Could you check a few things on this drawing? It's one solid part, dimensions in mm from its lowest x, y, z. A direction names the side the tool comes from. Coordinates: 2 decimals unless noted, no trailing zeros. Order: outer loops, then holes, each group sorted by start corner. A loop starts at its lowest first (then second) coordinate and runs counter-clockwise, first axis right, second up. Notation, with made-up numbers: (57.25, 73) - (111.25, 73) arc R32 cw to (111.25, 111) - close; hole circle Ø3 at (69, 32.25). An arc over 180 degrees is marked (long way). Return JSON: item names as keys, results as strings. Group by question number.
1) Imagine slicing it at A-A (y = 18). Write out the boundary of the cut face in (x, z).
2) For pin 1 Ø4 at (y, z) = (6, 75) entering from -X; pin 2 Ø3 at (x, y) = (9.5, 23) entering from -Z; pin 3 Ø1.2 at (x, y) = (9.5, 13.5) entering from -Z, each with a flat end and sliding along its axis, tell me the tip position at first contact or that it passes through.
3) If I drill on line 1 along Z through (x, y) = (28.5, 18.5); line 2 along X through (y, z) = (13, 24); line 3 along Z through (x, y) = (23, 21), over which ranges is the centre line in solid material (lowest first)?
4) Which directions (+Z, -Z, +X, -X, +Y, -Y) give clear straight access to the entire face, cutting with the end or side of a thin tool? Please do the marked faces 1 and 2.
5) Imagine slicing it at D-D (x = 4). Write out the boundary of the cut face in (y, z), and give its area (3 significant figures).
6) Imagine slicing it at B-B (z = 68). Write out the boundary of the cut face in (x, y).
7) Imagine slicing it at C-C (y = 27.5). Write out the boundary of the cut face in (x, z).
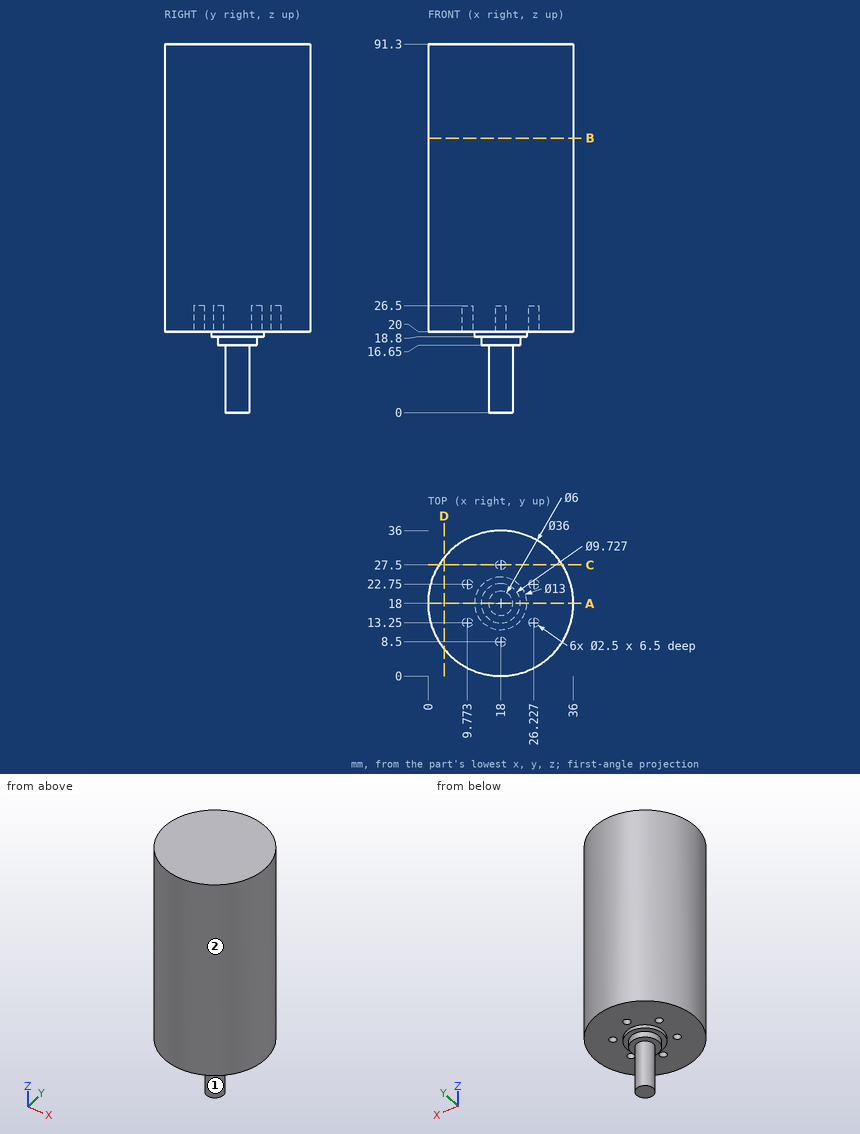
Calculated:
{
 "1": {"outline": "(0, 20) - (11.5, 20) - (11.5, 18.8) - (13.14, 18.8) - (13.14, 16.65) - (15, 16.65) - (15, 0) - (21, 0) - (21, 16.65) - (22.86, 16.65) - (22.86, 18.8) - (24.5, 18.8) - (24.5, 20) - (36, 20) - (36, 91.3) - (0, 91.3) - close"},
 "2": {"pin 1": "x = 3.03", "pin 2": "z = 20", "pin 3": "z = 26.5"},
 "3": {"line 1": "20 to 91.3", "line 2": "0.71 to 8.55, 11 to 25, 27.45 to 35.29", "line 3": "18.8 to 91.3"},
 "4": {"face 1": "-Z", "face 2": "+Z, -Z"},
 "5": {"outline": "(6.69, 20) - (29.31, 20) - (29.31, 91.3) - (6.69, 91.3) - close", "area": "1,610 mm2"},
 "6": {"outline": "circle Ø36 at (18, 18)"},
 "7": {"outline": "(2.71, 20) - (16.75, 20) - (16.75, 26.5) - (19.25, 26.5) - (19.25, 20) - (33.29, 20) - (33.29, 91.3) - (2.71, 91.3) - close"}
}
